from build123d import *

# Parameters (mm, degrees)
SKETCH1_W                                       = 35
SKETCH1_H                                       = 10
BOSS_EXTRUDE1_DEPTH                             = 8
CSK_FOR_M3_FLAT_HEAD_MACHINE_SCREW1_D           = 3.2
CSK_FOR_M3_FLAT_HEAD_MACHINE_SCREW1_CSINK_D     = 6.3
CSK_FOR_M3_FLAT_HEAD_MACHINE_SCREW1_CSINK_ANGLE = 90
SKETCH1_3_R                                     = 3.225
CUT_EXTRUDE2_DEPTH                              = 6.35
FILLET1_R                                       = 1


with BuildPart() as part:
    # Sketch1 → Boss-Extrude1 (new body)
    with BuildSketch(Plane(origin=(0, 0, 0), x_dir=(1, 0, 0), z_dir=(0, 1, 0))):
        Rectangle(SKETCH1_W, SKETCH1_H)
    extrude(amount=-BOSS_EXTRUDE1_DEPTH)

    # CSK for M3 Flat Head Machine Screw1 (through all)
    with Locations(Plane(origin=(-14, 0, 0), x_dir=(0, 0, 1), z_dir=(0, 1, 0))):
        with Locations((0, 0), (0, 28)):
            CounterSinkHole(CSK_FOR_M3_FLAT_HEAD_MACHINE_SCREW1_D / 2, CSK_FOR_M3_FLAT_HEAD_MACHINE_SCREW1_CSINK_D / 2, counter_sink_angle=CSK_FOR_M3_FLAT_HEAD_MACHINE_SCREW1_CSINK_ANGLE)

    # Sketch1_3 → Cut-Extrude2 (cut)
    with BuildSketch(Plane(origin=(0, 0, 0), x_dir=(1, 0, 0), z_dir=(0, 1, 0))):
        with Locations(Location((0, 0, 0), (0, 0, 270))):
            Circle(SKETCH1_3_R)
    extrude(amount=-CUT_EXTRUDE2_DEPTH, mode=Mode.SUBTRACT)

    # Fillet1
    fillet1_edges = [part.edges().sort_by_distance(p)[0] for p in [
        (-17.5, -4, -5),
        (17.5, -4, -5),
        (17.5, -4, 5),
        (-17.5, -4, 5),
    ]]
    fillet(fillet1_edges, radius=FILLET1_R)


solid = part.part
Source: CAD feature listing. Evaluate the final solid. Frame: model axes, mm. A direction names the side the tool comes from. Coordinates: 2 decimals unless noted, no trailing zeros. Loops run counter-clockwise (first coordinate to the right, second up) from the corner with the lowest first, then second, coordinate; pieces in that order, holes last. Notation, with made-up numbers: (78, -34) - (101, -34) arc R19 ccw to (101, -7) - close; hole circle Ø8 at (88, 25). An arc over 180 degrees is marked (long way). One line per item, written item: value. Start each with the question number.
1. Contact query for flat-ended pins moving along their axis: P1, Ø4, axis at x = -14, z = 0, coming from the +Y side; P2, Ø5, axis at x = 14, z = 0, coming from the +Y side; P3, Ø3, axis at x = -0.5, z = -0.5, coming from the +Y side. Output: stop coordinate, or through.
2. Set-up query: faces 1 (the flat face through (0, -6.35, 0)), 2 (the flat face through (-0.2, 0, -3.4)). Return all of +Z, -Z, +X, -X, +Y, -Y with unobstructed straight access to the full face (end or side cutting, diameter ignored); none if empty.
3. Section A-A (x = 14). Return the cut outline in (y, z), and give its area (3 significant figures).
4. Section B-B (z = 0). Return the cut outline in (x, y) (3 decimals).
5. Ray query, L1, parallel to X at y = -4.75, z = 0 (3 decimals); L2, parallel to X at y = -4, z = 0.5; L3, parallel to Z at x = 14, y = -5.5. Return the intervals inside material, ascending.
6. Section D-D (x = 0). Return the cut outline in (y, z) (3 decimals).
7. Mould query, pull axis X, two halves, no side actions, for faces 3 (the cylindrical face through (17.199, -4.056, -4.715)), 4 (the cylindrical face through (-12.414, -4.82, 0.208)), 5 (the flat face through (0, -4, 5)). Classes: pulls with the +X half, pulls with the -X half, needs draft (parallel to the pull), parting line crosses it, or undercut.
8. Section C-C (y = -6). Return the cut outline in (x, z) (3 decimals).
Verdict:
1. P1: stops at y = -1.15
1. P2: stops at y = -0.65
1. P3: stops at y = -6.35
2. face 1: +Y
2. face 2: +Z, -Z, +X, -X, +Y
3. outline: (-8, -5) - (0, -5) - (0, -3.15) - (-1.55, -1.6) - (-8, -1.6) - close; (-8, 1.6) - (-1.55, 1.6) - (0, 3.15) - (0, 5) - (-8, 5) - close
3. area: 52.0 mm2
4. outline: (-17.5, -8) - (-15.6, -8) - (-15.6, -1.55) - (-17.15, 0) - (-17.5, 0) - close; (-12.4, -8) - (12.4, -8) - (12.4, -1.55) - (10.85, 0) - (3.225, 0) - (3.225, -6.35) - (-3.225, -6.35) - (-3.225, 0) - (-10.85, 0) - (-12.4, -1.55) - close; (15.6, -8) - (17.5, -8) - (17.5, 0) - (17.15, 0) - (15.6, -1.55) - close
5. L1: x = -17.5 to -15.6, -12.4 to -3.225, 3.225 to 12.4, 15.6 to 17.5
5. L2: x = -17.5 to -15.52, -12.48 to -3.19, 3.19 to 12.48, 15.52 to 17.5
5. L3: z = -5 to -1.6, 1.6 to 5
6. outline: (-8, -5) - (0, -5) - (0, -3.225) - (-6.35, -3.225) - (-6.35, 3.225) - (0, 3.225) - (0, 5) - (-8, 5) - close
7. face 3: pulls with the +X half
7. face 4: undercut
7. face 5: needs draft
8. outline: (-17.5, -4) arc R1 ccw to (-16.5, -5) - (16.5, -5) arc R1 ccw to (17.5, -4) - (17.5, 4) arc R1 ccw to (16.5, 5) - (-16.5, 5) arc R1 ccw to (-17.5, 4) - close; hole circle Ø3.2 at (-14, 0); hole circle Ø6.45 at (0, 0); hole circle Ø3.2 at (14, 0)
